Part print with two shaded views. Sizes in mm from the minimum x, y, z corner. A direction names the side the tool comes from. Round coordinates to 2 decimals unless told otherwise and drop trailing zeros. Order: outer loops, then holes, each group sorted by start corner. A loop starts at its lowest first (then second) coordinate and runs counter-clockwise, first axis right, second up. Notation, with made-up numbers: M 48.25,65.25 L 69.25,65.25 A33 ccw 69.25,96.25 Z; hole C 5,70.25 d6. An arc over 180 degrees is marked long. Return JSON: item names as keys, results as strings. Group by question number.
Item 1: Pin check, flat tips, straight feed: pin 1 Ø2 at (x, y) = (16, 6) entering from +Z; pin 2 Ø4 at (y, z) = (2.5, 7) entering from -X; pin 3 Ø4 at (x, y) = (6, 4) entering from +Z. Stop position of each tip, or through.
Item 2: Probe line 1 along X through (y, z) = (1, 5.75); line 2 along X through (y, z) = (5.5, 9.75); line 3 along Z through (x, y) = (10.25, 6.5). List the from-to ranges inside material, lowest first.
Item 3: Slice it at A-A on x = 9.55. Write the cut outline in (y, z).
Item 4: Pull direction Z, two halves, no side cores. Call the marked faces 3, 4 and 5: pulls with the +Z half, pulls with the -Z half, needs draft (parallel to the pull), parting line crosses it, or undercut.
Item 5: Slice it at C-C on y = 6. Write the cut outline in (x, z), then the cut area to 3 significant figures.
Item 6: Slice it at D-D on z = 17.5. Write the cut outline in (x, y), then the cut area to 3 significant figures.
Item 7: Slice it at B-B on z = 9.55. Write the cut outline in (x, y), then the cut area to 3 significant figures.
Item 8: Which spindle directions (+Z, -Z, +X, -X, +Y, -Y) get a long thin tool onto all of the face, cutting with end or side? Do the marked faces 1 and 2. Say none if no direction does.
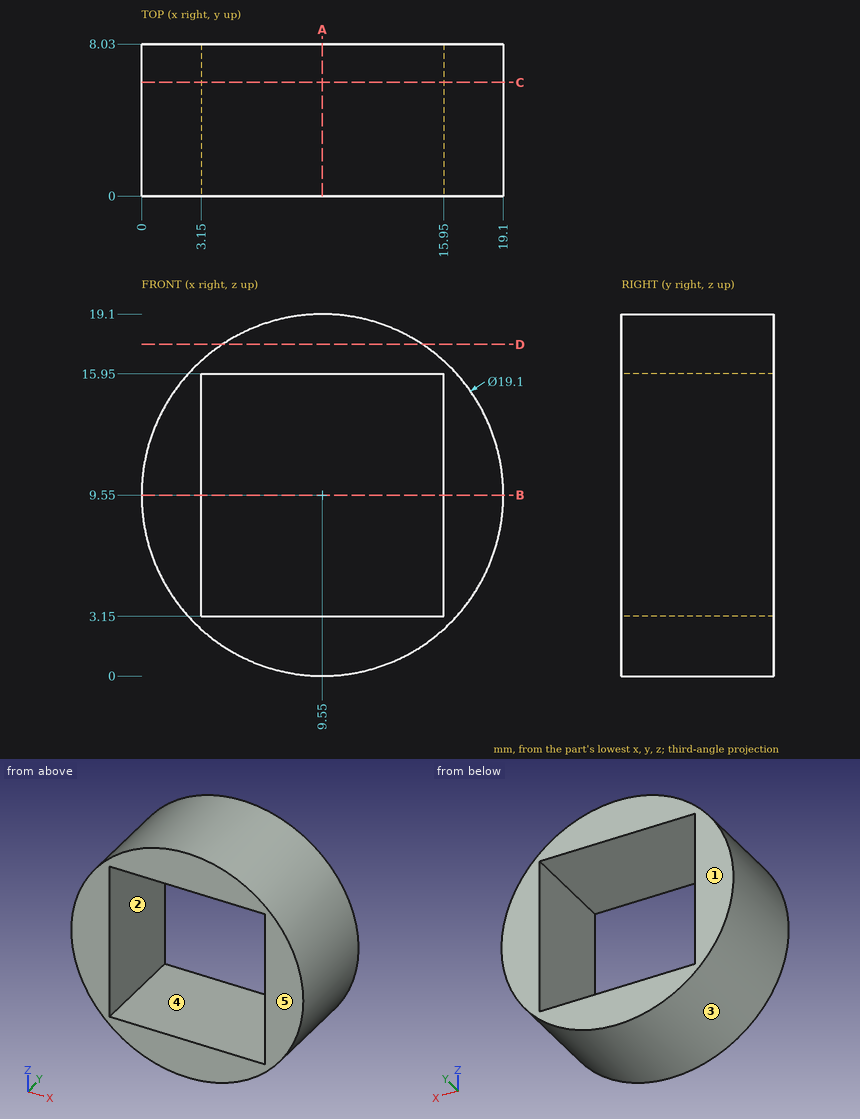
Output values:
{
 "1": {"pin 1": "z = 17.39", "pin 2": "x = 0.02", "pin 3": "z = 18.97"},
 "2": {"line 1": "0.79 to 3.15, 15.95 to 18.31", "line 2": "0 to 3.15, 15.95 to 19.1", "line 3": "0.03 to 3.15, 15.95 to 19.07"},
 "3": {"outline": "M 0,0 L 8.03,0 L 8.03,3.15 L 0,3.15 Z; M 0,15.95 L 8.03,15.95 L 8.03,19.1 L 0,19.1 Z"},
 "4": {"face 3": "parting line crosses it", "face 4": "undercut", "face 5": "needs draft"},
 "5": {"outline": "C 9.55,9.55 d19.1; hole M 3.15,3.15 L 15.95,3.15 L 15.95,15.95 L 3.15,15.95 Z", "area": "123 mm²"},
 "6": {"outline": "M 4.26,0 L 14.84,0 L 14.84,8.03 L 4.26,8.03 Z", "area": "85.0 mm²"},
 "7": {"outline": "M 0,0 L 3.15,0 L 3.15,8.03 L 0,8.03 Z; M 15.95,0 L 19.1,0 L 19.1,8.03 L 15.95,8.03 Z", "area": "50.6 mm²"},
 "8": {"face 1": "+Z, -Z, +X, -X, +Y", "face 2": "+Y, -Y"}
}
